For this review, take the finished solid that the model builds, in its own axes (mm). Give positions to 0.01 mm unless a question says otherwise; leave off trailing zeros. Loops run counter-clockwise (first coordinate to the right, second up) from the corner with the lowest first, then second, coordinate; pieces in that order, holes last. Notation, with made-up numbers: (-1, 56) -> (49, 56) arc R14 ccw to (49, 77) -> close; hole circle Ø4 at (8.25, -2). An arc over 180 degrees is marked (long way). Write each question's results on one line, items separated by ' | '. Start each with the question number.
```python
from build123d import *

# Parameters (mm, degrees)
ESQUISSE1_R        = 1.5
ESQUISSE1_R_2      = 3.8
ESQUISSE1_R_3      = 1.725
BOSS_EXTRU_1_DEPTH = 3


with BuildPart() as part:
    # Esquisse1 → Boss.-Extru.1 (new body)
    with BuildSketch(Plane.XY):
        with BuildLine():
            Line((19.21041076, -67.22505422), (26.66041076, -67.22505422))
            Line((26.66041076, -67.22505422), (26.66041076, 32.77494578))
            Line((26.66041076, 32.77494578), (46.66041076, 32.77494578))
            Line((46.66041076, 32.77494578), (46.66041076, -67.22505422))
            Line((46.66041076, -67.22505422), (99.16041076, -67.22505422))
            Line((99.16041076, -67.22505422), (99.16041076, 32.77494578))
            Line((99.16041076, 32.77494578), (119.16041076, 32.77494578))
            Line((119.16041076, 32.77494578), (119.16041076, -67.22505422))
            Line((119.16041076, -67.22505422), (171.66041076, -67.22505422))
            Line((171.66041076, -67.22505422), (171.66041076, 32.77494578))
            Line((171.66041076, 32.77494578), (189.66041076, 32.77494578))
            Line((189.66041076, 32.77494578), (189.66041076, 78.53494578))
            Line((189.66041076, 78.53494578), (183.66041076, 78.53494578))
            Line((183.66041076, 78.53494578), (183.66041076, 80.53494578))
            Line((183.66041076, 80.53494578), (194.78041076, 80.53494578))
            ThreePointArc((194.78041076, 80.53494578), (205.90041076, 91.65494578), (194.78041076, 102.77494578))
            Line((194.78041076, 102.77494578), (11.09041076, 102.77494578))
            ThreePointArc((11.09041076, 102.77494578), (-0.02958924, 91.65494578), (11.09041076, 80.53494578))
            Line((11.09041076, 80.53494578), (22.21041076, 80.53494578))
            Line((22.21041076, 80.53494578), (22.21041076, 78.53494578))
            Line((22.21041076, 78.53494578), (19.21041076, 78.53494578))
            Line((19.21041076, 78.53494578), (19.21041076, -67.22505422))
        make_face()
        with Locations((194.78041076, 91.65494578)):
            Circle(ESQUISSE1_R, mode=Mode.SUBTRACT)
        with Locations((11.09041076, 91.65494578)):
            Circle(ESQUISSE1_R_2, mode=Mode.SUBTRACT)
        with Locations((11.09041076, 99.26494578)):
            Circle(ESQUISSE1_R_3, mode=Mode.SUBTRACT)
        with Locations((18.70041076, 91.65494578)):
            Circle(ESQUISSE1_R_3, mode=Mode.SUBTRACT)
        with Locations((11.09041076, 84.04494578)):
            Circle(ESQUISSE1_R_3, mode=Mode.SUBTRACT)
        with Locations((3.48041076, 91.65494578)):
            Circle(ESQUISSE1_R_3, mode=Mode.SUBTRACT)
    extrude(amount=BOSS_EXTRU_1_DEPTH)


solid = part.part
```
1. Draft analysis for pull direction X (two halves, no side actions). For faces 1 (the cylindrical face through (10.267, 87.945, 1.479)), 2 (the flat face through (101, 38, 3)), 3 (the cylindrical face through (205.898, 91.41, 1.479)), 4 (the cylindrical face through (-0.027, 91.899, 1.479)), state which applies: released by +X, released by -X, zero draft, split by the parting line, or undercut.
2. For pin 1 Ø2 at (x, y) = (3.48, 91.65) entering from -Z; pin 2 Ø0.9 at (y, z) = (-6.5, 1.5) entering from -X; pin 3 Ø1.5 at (x, z) = (109, 1.5) entering from -Y; pin 4 Ø1.5 at (y, z) = (-48, 0.5) entering from +X, all flat-tipped, find the tip position at first contact; note any pin that passes through.
3. We need section C-C (x = 109). Write out the cut boundary in (y, z).
4. We need section A-A (y = 5). Write out the cut boundary in (x, z), plus the area to 3 significant figures.
5. We need section B-B (z = 1.9). Write out the cut boundary in (x, y) (3 decimals), plus the area to 3 significant figures.
6. Wall thickness on L1, parallel to X at y = 13.5, z = 1.5; L2, parallel to X at y = 77, z = 1.05; L3, parallel to X at y = 93, z = 0.4: over which ranges is each line inside the solid? List them lowest first.
7. We need section D-D (y = 67). Write out the cut boundary in (x, z).
Response:
1) face 1: undercut | face 2: zero draft | face 3: released by +X | face 4: released by -X
2) pin 1: passes through | pin 2: stops at x = 19.21 | pin 3: stops at y = 32.77 | pin 4: stops at x = 171.66
3) outline: (32.77, 0) -> (102.77, 0) -> (102.77, 3) -> (32.77, 3) -> close
4) outline: (19.21, 0) -> (26.66, 0) -> (26.66, 3) -> (19.21, 3) -> close; (46.66, 0) -> (99.16, 0) -> (99.16, 3) -> (46.66, 3) -> close; (119.16, 0) -> (171.66, 0) -> (171.66, 3) -> (119.16, 3) -> close | area: 337 mm2
5) outline: (11.09, 80.535) -> (22.21, 80.535) -> (22.21, 78.535) -> (19.21, 78.535) -> (19.21, -67.225) -> (26.66, -67.225) -> (26.66, 32.775) -> (46.66, 32.775) -> (46.66, -67.225) -> (99.16, -67.225) -> (99.16, 32.775) -> (119.16, 32.775) -> (119.16, -67.225) -> (171.66, -67.225) -> (171.66, 32.775) -> (189.66, 32.775) -> (189.66, 78.535) -> (183.66, 78.535) -> (183.66, 80.535) -> (194.78, 80.535) arc R11.12 ccw to (194.78, 102.775) -> (11.09, 102.775) arc R11.12 ccw to start; hole circle Ø3.45 at (3.48, 91.655); hole circle Ø7.6 at (11.09, 91.655); hole circle Ø3.45 at (11.09, 84.045); hole circle Ø3.45 at (11.09, 99.265); hole circle Ø3.45 at (18.7, 91.655); hole circle Ø3 at (194.78, 91.655) | area: 23,800 mm2
6) L1: x = 19.21 to 26.66, 46.66 to 99.16, 119.16 to 171.66 | L2: x = 19.21 to 189.66 | L3: x = 0.05 to 2.4, 4.56 to 7.54, 14.64 to 17.62, 19.78 to 194.12, 195.44 to 205.82
7) outline: (19.21, 0) -> (189.66, 0) -> (189.66, 3) -> (19.21, 3) -> close
